```python
from build123d import *

# Parameters (mm, degrees)
SKETCH1_R                            = 3.75
BOSS_EXTRUDE1_DEPTH                  = 35
SKETCH5_W                            = 11.25
SKETCH5_H                            = 102.5
CUT_EXTRUDE1_DEPTH                   = 121.441894704
F_3_2_3_2_DIAMETER_HOLE1_D           = 3.2
F_3_2_3_2_DIAMETER_HOLE1_CSINK_D     = 3.25
F_3_2_3_2_DIAMETER_HOLE1_CSINK_ANGLE = 90
CHAMFER1_SIZE                        = 2.5
FILLET1_R                            = 4


with BuildPart() as part:
    # Sketch1 → Boss-Extrude1 (new body)
    with BuildSketch(Plane.XY):
        with BuildLine():
            Line((0, 0), (-12.5, 0))
            Line((-12.5, 0), (-12.5, 100))
            ThreePointArc((-12.5, 100), (0, 112.5), (12.5, 100))
            Line((12.5, 100), (12.5, 0))
            Line((12.5, 0), (0, 0))
        make_face()
        with Locations((0, 100)):
            Circle(SKETCH1_R, mode=Mode.SUBTRACT)
    extrude(amount=BOSS_EXTRUDE1_DEPTH)

    # Sketch5 → Cut-Extrude1 (cut, through all)
    with BuildSketch(Plane(origin=(12.5, 0, 0), x_dir=(0, 0, -1), z_dir=(1, 0, 0))):
        with Locations((-29.375, 61.25)):
            Rectangle(SKETCH5_W, SKETCH5_H)
        with Locations((-5.625, 61.25)):
            Rectangle(SKETCH5_W, SKETCH5_H)
    extrude(amount=-CUT_EXTRUDE1_DEPTH, mode=Mode.SUBTRACT)

    # Ø3.2 (3.2) Diameter Hole1 (through all)
    with Locations(Plane(origin=(0, 10, 0), x_dir=(1, 0, 0), z_dir=(0, 1, 0))):
        with Locations((-7.5, -5.625), (7.5, -5.625), (7.5, -29.375), (-7.5, -29.375)):
            CounterSinkHole(F_3_2_3_2_DIAMETER_HOLE1_D / 2, F_3_2_3_2_DIAMETER_HOLE1_CSINK_D / 2, counter_sink_angle=F_3_2_3_2_DIAMETER_HOLE1_CSINK_ANGLE)

    # Chamfer1
    chamfer1_edges = [part.edges().sort_by_distance(p)[0] for p in [
        (-3.75, 100, 23.75),
    ]]
    chamfer(chamfer1_edges, length=CHAMFER1_SIZE)

    # Fillet1
    fillet1_edges = [part.edges().sort_by_distance(p)[0] for p in [
        (-3.75, 100, 21.25),
    ]]
    fillet(fillet1_edges, radius=FILLET1_R)


solid = part.part
```
Build history of the part. All positions in model axes, mm. A direction names the side the tool comes from. Coordinates: 2 decimals unless noted, no trailing zeros. Order: outer loops, then holes, each group sorted by start corner. A loop starts at its lowest first (then second) coordinate and runs counter-clockwise, first axis right, second up. Notation, with made-up numbers: M -17.75,-35 L 11.25,-35 A21 cw 11.25,-3 Z; hole C 40,-38.5 d9. An arc over 180 degrees is marked long. One line per question, with ' | ' between items. Start each with the question number.
1. Mould opens along Z. For faces 1 (the face through (-7.29, 4.92, 27.79)), 2 (the face through (0, 61, 23.75)), 3 (the face through (0, 10, 29)) say: +Z half, -Z half, draft (parallel to the pull), parting line (faces both ways), or undercut.
2. Flat gauge pins, fed straight in: P1, Ø9, axis at x = 3.5, z = 5.5, coming from the +Y side; P2, Ø2, axis at x = -9.5, z = 18.5, coming from the +Y side; P3, Ø3, axis at x = 7.5, z = 5.625, coming from the +Y side; P4, Ø6, axis at x = -9, y = 63.5, coming from the +Z side. Where does each tip first touch, or does it go through?
3. Cut at D-D (z = 10). Write the cut outline in (x, y).
4. Tool access for faces 4 (the face through (0, 61, 11.25)), 5 (the face through (-12.5, 38, 17)): list every direction of +Z, -Z, +X, -X, +Y, -Y with a clear straight run to the whole face (end or side of a thin tool).
5. Cut at A-A (z = 16). Write the cut outline in (x, y), plus the area to 3 significant figures.
6. Cut at C-C (y = 46.5). Write the cut outline in (x, z), plus the area to 4 significant figures.
7. Cut at B-B (x = 7.5). Write the cut outline in (y, z) (3 decimals), plus the area to 3 significant figures.
8. Wall check: line 1 along Z through (x, y) = (-7.5, 5.75) (3 decimals); line 2 along Z through (x, y) = (-1.75, 17); line 3 along X through (y, z) = (100, 17.5). Give the ranges that are in metal, low to high. Write a range as [from, to].
The answers:
1) face 1: undercut | face 2: +Z half | face 3: draft
2) P1: stops at y = 10 | P2: stops at y = 109.17 | P3: passes through | P4: stops at z = 23.75
3) outline: M -12.5,0 L 12.5,0 L 12.5,10 L -12.5,10 Z
4) face 4: -Z, +X, -X, +Y | face 5: +Z, -Z, -X, +Y, -Y
5) outline: M -12.5,0 L 12.5,0 L 12.5,100 A12.5 ccw -12.5,100 Z; hole C 0,100 d7.5 | area: 2,700 mm2
6) outline: M -12.5,11.25 L 12.5,11.25 L 12.5,23.75 L -12.5,23.75 Z | area: 312.5 mm2
7) outline: M 0,0 L 10,0 L 10,4 L 9.975,4.025 L 0,4.025 Z; M 0,7.225 L 9.975,7.225 L 10,7.25 L 10,11.25 L 110,11.25 L 110,23.75 L 10,23.75 L 10,27.75 L 9.975,27.775 L 0,27.775 Z; M 0,30.975 L 9.975,30.975 L 10,31 L 10,35 L 0,35 Z | area: 1,540 mm2
8) line 1: z = [0, 4.025], [7.225, 27.775], [30.975, 35] | line 2: z = [11.25, 23.75] | line 3: x = [-12.5, -3.75], [3.75, 12.5]
